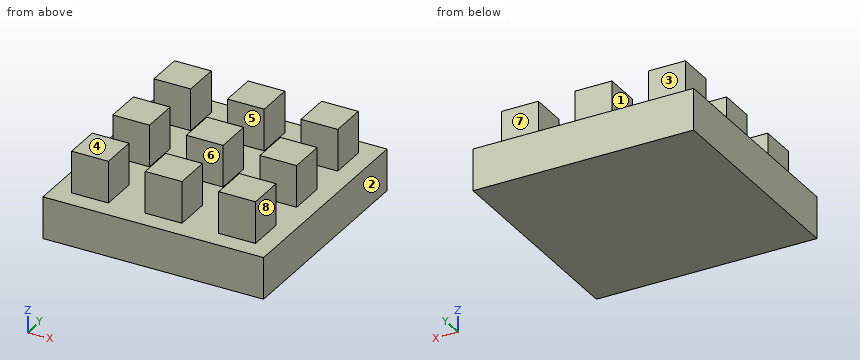
from build123d import *

# Parameters (mm, degrees)
F0_W     = 44
F0_H     = 44
F1_DEPTH = 50
F0_W_2   = 264
F0_H_2   = 264
F4_DEPTH = 50


with BuildPart() as f1:
    # F0 (on Top) → F1 (new body)
    with BuildSketch(Plane.XY):
        with Locations((-88, 0)):
            Rectangle(F0_W, F0_H)
    extrude(amount=F1_DEPTH)


with BuildPart() as f1b:
    # F0 (on Top) → F1, piece 2 (new body)
    with BuildSketch(Plane.XY):
        with Locations((-88, 88)):
            Rectangle(F0_W, F0_H)
    extrude(amount=F1_DEPTH)


with BuildPart() as f1c:
    # F0 (on Top) → F1, piece 3 (new body)
    with BuildSketch(Plane.XY):
        with Locations((0, 88)):
            Rectangle(F0_W, F0_H)
    extrude(amount=F1_DEPTH)


with BuildPart() as f1d:
    # F0 (on Top) → F1, piece 4 (new body)
    with BuildSketch(Plane.XY):
        Rectangle(F0_W, F0_H)
    extrude(amount=F1_DEPTH)


with BuildPart() as f2_1:
    # F2: instance of F1
    add(f1.part.mirror(Plane.YZ))


with BuildPart() as f2_2:
    # F2: instance of F1b
    add(f1b.part.mirror(Plane.YZ))


with BuildPart() as f3_1:
    # F3: instance of F1b
    add(f1b.part.mirror(Plane.XZ))


with BuildPart() as f3_2:
    # F3: instance of F1c
    add(f1c.part.mirror(Plane.XZ))


with BuildPart() as f3_3:
    # F3: instance of F2_2
    add(f2_2.part.mirror(Plane.XZ))


with BuildPart() as f1_1:
    add(f1.part)

    add(f1b.part)  # F4 merges F1b

    add(f1c.part)  # F4 merges F1c

    add(f1d.part)  # F4 merges F1d

    add(f2_1.part)  # F4 merges F2_1

    add(f2_2.part)  # F4 merges F2_2

    add(f3_1.part)  # F4 merges F3_1

    add(f3_2.part)  # F4 merges F3_2

    add(f3_3.part)  # F4 merges F3_3
    # F0 (on Top) → F4 (join)
    with BuildSketch(Plane.XY):
        Rectangle(F0_W_2, F0_H_2)
        with Locations((-88, 0)):
            Rectangle(F0_W, F0_H, mode=Mode.SUBTRACT)
        with Locations((-88, 88)):
            Rectangle(F0_W, F0_H, mode=Mode.SUBTRACT)
        Rectangle(F0_W, F0_H, mode=Mode.SUBTRACT)
        with Locations((0, 88)):
            Rectangle(F0_W, F0_H, mode=Mode.SUBTRACT)
        with Locations((-88, 0)):
            Rectangle(F0_W, F0_H)
        Rectangle(F0_W, F0_H)
        with Locations((-88, 88)):
            Rectangle(F0_W, F0_H)
        with Locations((0, 88)):
            Rectangle(F0_W, F0_H)
    extrude(amount=-F4_DEPTH)


solid = f1_1.part
Geometry check sheet. Reference: the model listing, model coordinates, mm. Face numbers are marked on the shaded views. A direction names the side the tool comes from. Round coordinates to 2 decimals unless told otherwise and drop trailing zeros. Write each loop counter-clockwise with the first axis right and the second up, starting at its lowest first coordinate (ties: lowest second). Pieces come first, ordered by that corner, then holes.
Item 1: Mould release check, pull along Y, two halves, no side actions. Record for the marked faces 6, 7 and 8: +Y half, -Y half, draft (parallel to the pull), parting line (faces both ways), or undercut.
Determined:
face 6: undercut
face 7: +Y half
face 8: draft
Item 2: Material ranges on line 1 along X through (y, z) = (-3.5, 17); line 2 along Z through (x, y) = (53.5, 113), recorded low to high.
Determined:
line 1: x = -110 to -66, -22 to 22, 66 to 110
line 2: z = -50 to 0
Item 3: Section check B-B (z = 12). Give the number of separate pieces and of enclosed holes in the cut face, plus the area to 3 significant figures.
Determined:
separate pieces: 9
enclosed holes: 0
area: 17,400 mm2
Item 4: Section check A-A (x = 103.5). Record the boundary of the cut face in (y, z), plus the area to 3 significant figures.
Determined:
outline: (-132, -50) - (132, -50) - (132, 0) - (110, 0) - (110, 50) - (66, 50) - (66, 0) - (22, 0) - (22, 50) - (-22, 50) - (-22, 0) - (-66, 0) - (-66, 50) - (-110, 50) - (-110, 0) - (-132, 0) - close
area: 19,800 mm2
Item 5: Access from +Z, -Z, +X, -X, +Y, -Y to the whole of each face (thin tool, end or side, straight path). Record for the marked faces 1, 2, 3, 4 and 5.
Determined:
face 1: +Z, +Y, -Y
face 2: +Z, -Z, +X, +Y, -Y
face 3: +Z, +X, -X, +Y
face 4: +Z, +X, -X, +Y, -Y
face 5: +Z, +X, -X
Item 6: Section check C-C (y = 53). Record the boundary of the cut face in (x, z), plus the area to 3 significant figures.
Determined:
outline: (-132, -50) - (132, -50) - (132, 0) - (-132, 0) - close
area: 13,200 mm2
Item 7: Go/stop test with flat-tipped pins: pin 1 Ø12 at (x, y) = (-77, 53) entering from +Z; pin 2 Ø22 at (y, z) = (10.5, 21.5) entering from -X; pin 3 Ø2 at (y, z) = (-84.5, 33) entering from +X. Record where each tip stops, or that it passes through.
Determined:
pin 1: stops at z = 0
pin 2: stops at x = -110
pin 3: stops at x = 110
